Can you work these out from the model? Positions are in its coordinate system, mm. Face numbers are marked on the shaded views. A direction names the side the tool comes from. Give positions to 0.01 mm unless a question says otherwise; leave off trailing zeros. Order: outer loops, then holes, each group sorted by start corner. A loop starts at its lowest first (then second) coordinate and runs counter-clockwise, first axis right, second up. Notation, with made-up numbers: (14.5, 26.25) -> (71.5, 26.25) arc R19 cw to (71.5, 30.25) -> close; hole circle Ø5 at (61, 59). An arc over 180 degrees is marked (long way). Answer as a JSON object with one key per item and string values.
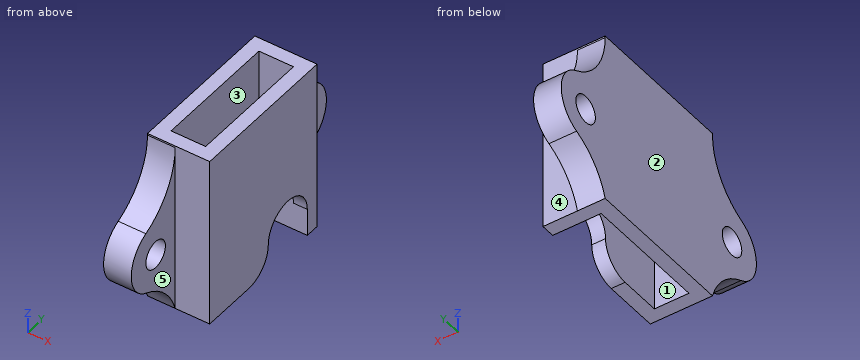
```python
from build123d import *

# Parameters (mm, degrees)
ESQUISSE1_W             = 9
ESQUISSE1_H             = 22
ESQUISSE1_W_2           = 5
ESQUISSE1_H_2           = 18
BOSS_EXTRU_1_DEPTH      = 25
ESQUISSE2_R             = 2
BOSS_EXTRU_2_DEPTH      = 4
CONG_1_R                = 10
ESQUISSE3_W             = 8
ESQUISSE3_H             = 8
ENL_V_MAT_EXTRU_1_DEPTH = 39.923000912
CONG_2_R                = 4


# Some blends are built 0.0001 mm under size
with BuildPart() as part:
    # Esquisse1 → Boss.-Extru.1 (new body)
    with BuildSketch(Plane.XY):
        with Locations((2.5, 9)):
            Rectangle(ESQUISSE1_W, ESQUISSE1_H)
        with Locations((2.5, 9)):
            Rectangle(ESQUISSE1_W_2, ESQUISSE1_H_2, mode=Mode.SUBTRACT)
    extrude(amount=BOSS_EXTRU_1_DEPTH)

    # Esquisse2 → Boss.-Extru.2 (add)
    # profile 1 of 2: a face of its own
    with BuildSketch(Plane.ZY.offset(2)):
        with BuildLine():
            Line((6, -2), (6, -6))
            ThreePointArc((6, -6), (11, -11), (16, -6))
            Line((16, -6), (16, -2))
            Line((16, -2), (6, -2))
        make_face()
        with Locations((11, -6)):
            Circle(ESQUISSE2_R, mode=Mode.SUBTRACT)
    # profile 2 of 2: a face of its own
    with BuildSketch(Plane.ZY.offset(2)):
        with BuildLine():
            Line((6, 20), (6, 24))
            ThreePointArc((6, 24), (11, 29), (16, 24))
            Line((16, 24), (16, 20))
            Line((16, 20), (6, 20))
        make_face()
        with Locations((11, 24)):
            Circle(ESQUISSE2_R, mode=Mode.SUBTRACT)
    extrude(amount=-BOSS_EXTRU_2_DEPTH)

    # Congé1
    # the kernel refuses this fillet: 10 mm, written as the material it adds along each edge
    with BuildSketch(Plane(origin=(-2, -2, 16), x_dir=(0, 0, 1), z_dir=(1, 0, 0))) as cong_1_piece_1:
        with BuildLine():
            CenterArc((8.747727085, 10), CONG_1_R, 203.578178478, 66.421821522)
            Line((-0.417424305, 6), (-1.333939444, 5.6))
            ThreePointArc((-1.333939444, 5.6), (-1, 4), (-1, 0))
            Line((-1, 0), (0, -1))
            Line((0, -1), (8.747727085, -1))
            Line((8.747727085, -1), (8.747727085, 0))
        make_face()
    extrude(amount=4)
    with BuildSketch(Plane(origin=(-2, 20, 16), x_dir=(0, 0, 1), z_dir=(1, 0, 0))) as cong_1_piece_2:
        with BuildLine():
            CenterArc((8.747727085, -10), CONG_1_R, 90, 66.421821522)
            Line((-0.417424305, -6), (-1.333939444, -5.6))
            ThreePointArc((-1.333939444, -5.6), (-1, -4), (-1, 0))
            Line((-1, 0), (0, 1))
            Line((0, 1), (8.747727085, 1))
            Line((8.747727085, 1), (8.747727085, 0))
        make_face()
    extrude(amount=4)
    with BuildSketch(Plane(origin=(-2, -2, 6), x_dir=(0, 0, -1), z_dir=(1, 0, 0))) as cong_1_piece_3:
        with BuildLine():
            CenterArc((8.931185798, -9.560760944), CONG_1_R, 107.044753414, 51.195378821)
            Line((-0.356271401, -5.853586981), (-1.285017121, -5.482869585))
            ThreePointArc((-1.285017121, -5.482869585), (-1, -4), (-1, 0))
            Line((-1, 0), (0, 1))
            ThreePointArc((0, 1), (3, 1), (5.70688142, 0.956076094))
            Line((5.70688142, 0.956076094), (6, 0))
        make_face()
    extrude(amount=4)
    with BuildSketch(Plane(origin=(-2, 20, 6), x_dir=(0, 0, -1), z_dir=(1, 0, 0))) as cong_1_piece_4:
        with BuildLine():
            CenterArc((8.931185798, 9.560760944), CONG_1_R, 201.759867765, 51.195378821)
            Line((-0.356271401, 5.853586981), (-1.285017121, 5.482869585))
            ThreePointArc((-1.285017121, 5.482869585), (-1, 4), (-1, 0))
            Line((-1, 0), (0, -1))
            ThreePointArc((0, -1), (3, -1), (5.70688142, -0.956076094))
            Line((5.70688142, -0.956076094), (6, 0))
        make_face()
    extrude(amount=4)

    # Esquisse3 → Enlèv. mat.-Extru.1 (cut, through all)
    with BuildSketch(Plane(origin=(0, 0, 0), x_dir=(0, 0, -1), z_dir=(1, 0, 0))):
        with Locations((-4, 14)):
            Rectangle(ESQUISSE3_W, ESQUISSE3_H)
    extrude(amount=ENL_V_MAT_EXTRU_1_DEPTH, mode=Mode.SUBTRACT)

    # Congé2
    cong_2_edges = [part.edges().sort_by_distance(p)[0] for p in [
        (6, 10, 0),
        (6, 10, 8),
        (6, 18, 8),
    ]]
    fillet(cong_2_edges, radius=CONG_2_R - 0.0001)  # a hair under: the kernel refuses the full size


solid = part.part
```
1. If we mould it in two halves opening along X, with no side actions, what happens to the marked faces 3, 4 and 5? For each: +X half, -X half, draft (parallel to the pull), parting line (faces both ways), or undercut.
Worked answers:
{"face 3": "undercut", "face 4": "draft", "face 5": "+X half"}
2. If we section it at A-A on z = 11: Please give me the cut outline in (x, y).
Worked answers:
{"outline": "(-2, -11) -> (2, -11) -> (2, -8) -> (-2, -8) -> close; (-2, -4) -> (2, -4) -> (2, -2) -> (7, -2) -> (7, 20) -> (2, 20) -> (2, 22) -> (-2, 22) -> close; (-2, 26) -> (2, 26) -> (2, 29) -> (-2, 29) -> close; hole (0, 0) -> (5, 0) -> (5, 18) -> (0, 18) -> close"}
3. If we section it at C-C on y = 2: Please give me the cut outline in (x, z).
Worked answers:
{"outline": "(-2, 0) -> (0, 0) -> (0, 25) -> (-2, 25) -> close; (5, 0) -> (7, 0) -> (7, 25) -> (5, 25) -> close"}
4. Please list where these lines run through material, in increasing order: L1, parallel to Y at x = 0.45, z = 11; L2, parallel to Y at x = -0.5, z = 11; L3, parallel to X at y = 0.5, z = 8.5.
Worked answers:
{"L1": "-11 to -8, -4 to 0, 18 to 22, 26 to 29", "L2": "-11 to -8, -4 to 22, 26 to 29", "L3": "-2 to 0, 5 to 7"}
5. If we section it at D-D on x = 0.5: Please give me the cut outline in (y, z).
Worked answers:
{"outline": "(-8, 15.58) arc R5 ccw to (-7.85, 6.36) arc R10 cw to (-2, 0) -> (0, 0) -> (0, 25) -> (-2, 25) -> (-2, 24.75) arc R10 cw to start; (18, 0) -> (20, 0) arc R10 cw to (25.85, 6.36) arc R5 ccw to (26, 15.58) arc R10 cw to (20, 24.75) -> (20, 25) -> (18, 25) -> close; hole circle Ø4 at (-6, 11); hole circle Ø4 at (24, 11)"}
6. Will these pins go through, and if not, where does the flat tip stop? pin 1 Ø2.5 at (x, z) = (2, 17.5) entering from +Y; pin 2 Ø7 at (y, z) = (-8.5, 6.5) entering from +X; pin 3 Ø1 at (x, z) = (-0.5, 13.5) entering from -Y.
Worked answers:
{"pin 1": "y = 24.73", "pin 2": "x = 2", "pin 3": "y = -10.58"}
7. If we section it at B-B on x = 3.5: Please give me the cut outline in (y, z).
Worked answers:
{"outline": "(-2, 0) -> (0, 0) -> (0, 25) -> (-2, 25) -> close; (18, 0) -> (20, 0) -> (20, 25) -> (18, 25) -> close"}
8. For the marked faces 1 and 2, which set-ups out of +Z, -Z, +X, -X, +Y, -Y let a thin tool reach every point of the face, with its end or its side?
Worked answers:
{"face 1": "+Z, -Z", "face 2": "+Z, -Z, -X, +Y, -Y"}
